Check sheet for the modelled part. Datum: model origin and axes. Units: mm. A direction names the side the tool comes from. Give positions to 0.01 mm unless a question says otherwise; leave off trailing zeros. Write each loop counter-clockwise with the first axis right and the second up, starting at its lowest first coordinate (ties: lowest second). Pieces come first, ordered by that corner, then holes.
from build123d import *

# Parameters (mm, degrees)
ESQUISSE1_W             = 30
ESQUISSE1_H             = 18
BOSS_EXTRU_1_DEPTH      = 8
ENL_V_MAT_EXTRU_1_DEPTH = 9
ENL_V_MAT_EXTRU_2_DEPTH = 4.2
CHANFREIN1_SIZE         = 18
CHANFREIN1_SIZE2        = 6.551464217
CHANFREIN1_PART_2_SIZE  = 18
CHANFREIN1_PART_2_SIZE2 = 6.551464217
CONG_1_R                = 2
ESQUISSE4_W             = 2.6
ESQUISSE4_H             = 5.2
ENL_V_MAT_EXTRU_3_DEPTH = 9
ESQUISSE5_R             = 1
ENL_V_MAT_EXTRU_4_DEPTH = 16
ESQUISSE6_W             = 6
ESQUISSE6_H             = 5.5
ESQUISSE6_R             = 1.7
BOSS_EXTRU_2_DEPTH      = 1.6


with BuildPart() as part:
    # Esquisse1 → Boss.-Extru.1 (new body)
    with BuildSketch(Plane.XY):
        with Locations((7, 0)):
            Rectangle(ESQUISSE1_W, ESQUISSE1_H)
    extrude(amount=BOSS_EXTRU_1_DEPTH)

    # Esquisse2 → Enlèv. mat.-Extru.1 (cut, through all)
    with BuildSketch(Plane.XY.offset(8)):
        with BuildLine():
            Line((-3, 2.2), (7, 2.2))
            ThreePointArc((7, 2.2), (9.2, 0), (7, -2.2))
            Line((7, -2.2), (-3, -2.2))
            ThreePointArc((-3, -2.2), (-5.2, 0), (-3, 2.2))
        make_face()
    extrude(amount=-ENL_V_MAT_EXTRU_1_DEPTH, mode=Mode.SUBTRACT)

    # Esquisse3 → Enlèv. mat.-Extru.2 (cut)
    with BuildSketch(Plane.XY.offset(8)):
        with BuildLine():
            Line((-3, 4), (7, 4))
            ThreePointArc((7, 4), (11, 0), (7, -4))
            Line((7, -4), (-3, -4))
            ThreePointArc((-3, -4), (-7, 0), (-3, 4))
        make_face()
    extrude(amount=-ENL_V_MAT_EXTRU_2_DEPTH, mode=Mode.SUBTRACT)

    # Chanfrein1
    chanfrein1_edges = [part.edges().sort_by_distance(p)[0] for p in [
        (-8, 9, 4),
    ]]
    chanfrein1_side = [part.faces().sort_by_distance(p)[0] for p in [
        (7, 9, 4),
    ]]
    chamfer(chanfrein1_edges, length=CHANFREIN1_SIZE, length2=CHANFREIN1_SIZE2, reference=chanfrein1_side[0])

    # Chanfrein1 part 2
    chanfrein1_part_2_edges = [part.edges().sort_by_distance(p)[0] for p in [
        (-8, -9, 4),
    ]]
    chanfrein1_part_2_side = [part.faces().sort_by_distance(p)[0] for p in [
        (7, -9, 4),
    ]]
    chamfer(chanfrein1_part_2_edges, length=CHANFREIN1_PART_2_SIZE, length2=CHANFREIN1_PART_2_SIZE2, reference=chanfrein1_part_2_side[0])

    # Congé1
    cong_1_edges = [part.edges().sort_by_distance(p)[0] for p in [
        (10, -9, 4),
        (-8, 2.448535783, 4),
        (-8, -2.448535783, 4),
        (10, 9, 4),
    ]]
    fillet(cong_1_edges, radius=CONG_1_R)

    # Esquisse4 → Enlèv. mat.-Extru.3 (cut, through all)
    with BuildSketch(Plane(origin=(0, 0, 0), x_dir=(-1, 0, 0), z_dir=(0, 0, -1))):
        with Locations((-17.7, -3.05)):
            Rectangle(ESQUISSE4_W, ESQUISSE4_H)
        with Locations((-17.7, 3.05)):
            Rectangle(ESQUISSE4_W, ESQUISSE4_H)
    extrude(amount=-ENL_V_MAT_EXTRU_3_DEPTH, mode=Mode.SUBTRACT)

    # Esquisse5 → Enlèv. mat.-Extru.4 (cut)
    with BuildSketch(Plane(origin=(22, 0, 0), x_dir=(0, 0, -1), z_dir=(1, 0, 0))):
        with Locations((-3, 3.25)):
            Circle(ESQUISSE5_R)
        with Locations((-3, -3.25)):
            Circle(ESQUISSE5_R)
    extrude(amount=-ENL_V_MAT_EXTRU_4_DEPTH, mode=Mode.SUBTRACT)

    # Esquisse6 → Boss.-Extru.2 (add)
    with BuildSketch(Plane(origin=(22, 0, 0), x_dir=(0, 0, -1), z_dir=(1, 0, 0))):
        with Locations((-3, -3.25)):
            Rectangle(ESQUISSE6_W, ESQUISSE6_H)
        with Locations((-3, -3.25)):
            Circle(ESQUISSE6_R, mode=Mode.SUBTRACT)
        with Locations((-3, 3.25)):
            Rectangle(ESQUISSE6_W, ESQUISSE6_H)
        with Locations((-3, 3.25)):
            Circle(ESQUISSE6_R, mode=Mode.SUBTRACT)
    extrude(amount=BOSS_EXTRU_2_DEPTH)


solid = part.part
1) Sectioned sample at C-C on x = 21. Record the boundary of the cut face in (y, z), then the cut area to 3 significant figures.
2) Draft check along X on faces 1 (the flat face through (2, 2.2, 2)), 2 (the cylindrical face through (-7.65, -2.18, 4.06)), 3 (the cylindrical face through (22.79, -3.9, 1.43)), 4 (the flat face through (19, -2.5, 3.9)). Enter one of: +X half, -X half, draft (parallel to the pull), parting line (faces both ways), or undercut.
3) Access from +Z, -Z, +X, -X, +Y, -Y to the whole of each face (thin tool, end or side, straight path). Record for faces 5 (the cylindrical face through (11.273, -3.633, 2.076)), 6 (the flat face through (23, -0.5, 3)), 7 (the cylindrical face through (9.2, 0, 1.9)).
4) Scan lines: L1, parallel to Y at x = 20.25, z = 3; L2, parallel to Y at x = 22.8, z = 3; L3, parallel to Z at x = 15.5, y = 3.25. Record each from-to range of solid material in increasing order.
5) Sectioned sample at A-A on y = 0. Record the boundary of the cut face in (x, z), then the cut area to 3 significant figures.
6) Gauge pin test, flat ends, axial feed: pin 1 (2.5 mm diameter, centred on y = 3.25, z = 3, fed in from +X); pin 2 (1.6 mm diameter, centred on y = -3.25, z = 3, fed in from -X); pin 3 (4.5 mm diameter, centred on y = -3.25, z = 3, fed in from -X); pin 4 (3.5 mm diameter, centred on x = 2, z = 6.5, fed in from -Y). Record the tip position at first contact, or that the pin passes through.
7) Sectioned sample at B-B on z = 7. Record the boundary of the cut face in (x, y).
8) Sectioned sample at D-D on x = 2. Record the boundary of the cut face in (y, z), then the cut area to 3 significant figures.
Answers below:
1. outline: (-9, 0) - (9, 0) - (9, 8) - (-9, 8) - close; hole circle Ø2 at (-3.25, 3); hole circle Ø2 at (3.25, 3)
1. area: 138 mm2
2. face 1: undercut
2. face 2: -X half
2. face 3: draft
2. face 4: undercut
3. face 5: +X
3. face 6: +Z, -Z, +X
3. face 7: +Z, -Z
4. L1: y = -9 to -4.25, -2.25 to 2.25, 4.25 to 9
4. L2: y = -6 to -4.95, -1.55 to -0.5, 0.5 to 1.55, 4.95 to 6
4. L3: z = 0 to 2, 4 to 8
5. outline: (-8, 0) - (-5.2, 0) - (-5.2, 3.8) - (-7, 3.8) - (-7, 8) - (-8, 8) - close; (9.2, 0) - (22, 0) - (22, 8) - (11, 8) - (11, 3.8) - (9.2, 3.8) - close
5. area: 110 mm2
6. pin 1: stops at x = 22
6. pin 2: stops at x = -7.43
6. pin 3: stops at x = -8
6. pin 4: stops at y = -6.73
7. outline: (-8, -1.05) arc R2 ccw to (-6.68, -2.93) - (9.67, -8.88) arc R2 ccw to (10.35, -9) - (22, -9) - (22, 9) - (10.35, 9) arc R2 ccw to (9.67, 8.88) - (-6.68, 2.93) arc R2 ccw to (-8, 1.05) - close; hole (-3, -4) - (7, -4) arc R4 ccw to (7, 4) - (-3, 4) arc R4 ccw to start; hole (16.4, -5.65) - (19, -5.65) - (19, -0.45) - (16.4, -0.45) - close; hole (16.4, 0.45) - (19, 0.45) - (19, 5.65) - (16.4, 5.65) - close
8. outline: (-6.09, 0) - (-2.2, 0) - (-2.2, 3.8) - (-4, 3.8) - (-4, 8) - (-6.09, 8) - close; (2.2, 0) - (6.09, 0) - (6.09, 8) - (4, 8) - (4, 3.8) - (2.2, 3.8) - close
8. area: 47.1 mm2
